For this review, take the finished solid that the model builds, in its own axes (mm). Coordinates: 2 decimals unless noted, no trailing zeros. Loops run counter-clockwise (first coordinate to the right, second up) from the corner with the lowest first, then second, coordinate; pieces in that order, holes last. Notation, with made-up numbers: M -21.5,51 L -13.5,51 A11 ccw -13.5,63 Z; hole C 35.5,44 d1. An arc over 180 degrees is marked long. Write item = value, one per line.
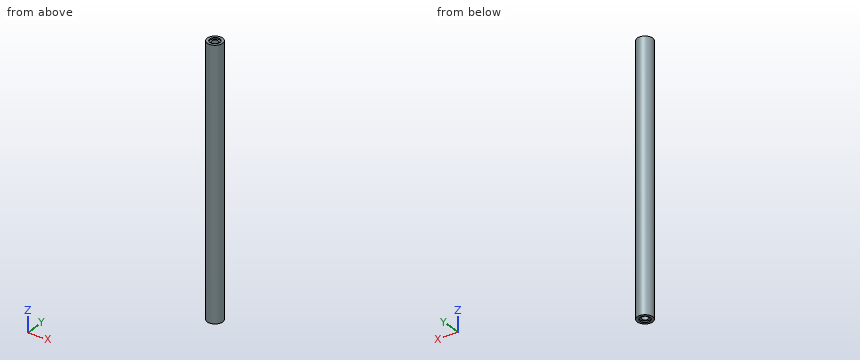
from build123d import *

# Parameters (mm, degrees)
SKETCH1_R                   = 9.525
BOSS_EXTRUDE1_DEPTH         = 327.025
SKETCH2_R                   = 6.3754
CUT_EXTRUDE1_DEPTH          = 1.524
F_3_8_16_TAPPED_HOLE1_D     = 7.9375
F_3_8_16_TAPPED_HOLE1_DEPTH = 25.4
F_3_8_16_TAPPED_HOLE1_TIP   = 2.384665582
CUT_EXTRUDE2_START          = -1.524
SKETCH5_R                   = 6.3754
CUT_EXTRUDE2_DEPTH          = 1.524
F_3_8_16_TAPPED_HOLE2_D     = 7.9375
F_3_8_16_TAPPED_HOLE2_DEPTH = 25.4
F_3_8_16_TAPPED_HOLE2_TIP   = 2.384665582


with BuildPart() as part:
    # Sketch1 → Boss-Extrude1 (new body)
    with BuildSketch(Plane.XY):
        with Locations(Location((0, 0, 0), (0, 0, 180))):
            Circle(SKETCH1_R)
    extrude(amount=BOSS_EXTRUDE1_DEPTH)

    # Sketch2 → Cut-Extrude1 (cut)
    with BuildSketch(Plane.XY.offset(327.025)):
        Circle(SKETCH2_R)
    extrude(amount=-CUT_EXTRUDE1_DEPTH, mode=Mode.SUBTRACT)

    # 3/8-16 Tapped Hole1
    with Locations(Plane.XY.offset(325.501)):
        with Locations((0, 0)):
            Hole(F_3_8_16_TAPPED_HOLE1_D / 2, depth=F_3_8_16_TAPPED_HOLE1_DEPTH)
            with Locations((0, 0, -(F_3_8_16_TAPPED_HOLE1_DEPTH + F_3_8_16_TAPPED_HOLE1_TIP / 2))):  # 118° drill point
                Cone(0, F_3_8_16_TAPPED_HOLE1_D / 2, F_3_8_16_TAPPED_HOLE1_TIP, mode=Mode.SUBTRACT)

    # Sketch5 → Cut-Extrude2 (cut)
    with BuildSketch(Plane(origin=(0, 0, 0), x_dir=(-1, 0, 0), z_dir=(0, 0, -1)).offset(CUT_EXTRUDE2_START)):
        with Locations(Location((0, 0, 0), (0, 0, 180))):
            Circle(SKETCH5_R)
    extrude(amount=CUT_EXTRUDE2_DEPTH, mode=Mode.SUBTRACT)

    # 3/8-16 Tapped Hole2
    with Locations(Plane(origin=(0, 0, 1.524), x_dir=(-1, 0, 0), z_dir=(0, 0, -1))):
        with Locations((0, 0)):
            Hole(F_3_8_16_TAPPED_HOLE2_D / 2, depth=F_3_8_16_TAPPED_HOLE2_DEPTH)
            with Locations((0, 0, -(F_3_8_16_TAPPED_HOLE2_DEPTH + F_3_8_16_TAPPED_HOLE2_TIP / 2))):  # 118° drill point
                Cone(0, F_3_8_16_TAPPED_HOLE2_D / 2, F_3_8_16_TAPPED_HOLE2_TIP, mode=Mode.SUBTRACT)


solid = part.part
Q1. Add section A-A (z = 145.5). Write out the cut boundary in (x, y) (3 decimals), and give its area (3 significant figures).
Solved:
outline = C 0,0 d19.05
area = 285 mm²
Q2. For pin 1 Ø3 at (y, z) = (-6, 219) entering from -X (3 decimals); pin 2 Ø5 at (x, z) = (-2, 182.5) entering from -Y (3 decimals); pin 3 Ø7 at (x, y) = (0, 0) entering from -Z; pin 4 Ø3 at (x, y) = (3.5, 0) entering from -Z, all flat-tipped, find the tip position at first contact; note any pin that passes through.
Solved:
pin_1 = -8.395
pin_2 = -9.525
pin_3 = 27.21
pin_4 = 1.52
Q3. For line 1 along Y through (x, z) = (0, 309.5) (3 decimals); line 2 along Y through (x, z) = (0, 326.5) (3 decimals); line 3 along Y through (x, z) = (1, 91.5), list the stretches that pass through material, from the lowest coordinate up.
Solved:
line_1 = -9.525 to -3.969, 3.969 to 9.525
line_2 = -9.525 to -6.375, 6.375 to 9.525
line_3 = -9.47 to 9.47
